Input: part model. Units: mm. Frame: model coordinates. A direction names the side the tool comes from. Give positions to 0.01 mm unless a question says otherwise; leave off trailing zeros. Write each loop counter-clockwise with the first axis right and the second up, starting at its lowest first coordinate (ties: lowest second). Pieces come first, ordered by that corner, then holes. Notation, with made-up numbers: (44.25, 87.5) -> (96.25, 87.5) arc R28 cw to (96.25, 122.5) -> close; hole circle Ø4 at (27, -24.5). An arc over 180 degrees is marked (long way). Return JSON: item names as keys, results as strings. Group by question number.
Item 1: Set-up query: faces 1 (the face through (-16, 16, -2)), 2 (the face through (0, 45, 0)), 3 (the face through (-12, 17, 4)), 4 (the face through (0, -12, 7)). Return all of +Z, -Z, +X, -X, +Y, -Y with unobstructed straight access to the full face (end or side cutting, diameter ignored); none if empty.
Item 2: Mould query, pull axis Z, two halves, no side actions, for faces 5 (the face through (16, 16, -2)), 6 (the face through (14.03, 21.27, 5)), 7 (the face through (0, 45, 7)), 8 (the face through (-14.028, 21.495, 3.72)). Classes: released by +Z, released by -Z, zero draft, split by the parting line, or undercut.
Item 3: Section A-A, the plane y = 0. Return loops of the section in (x, z), then the cut area to 3 significant figures.
Item 4: Section D-D, the plane y = 33. Return loops of the section in (x, z).
Item 5: Line query: line 1 (X direction, y = 0, z = 1.75); line 2 (Y direction, x = -4.5, z = 2.5); line 3 (Y direction, x = -15, z = 5.75). Output: solid intervals per line, ascending. Write a range as [from, to].
Item 6: Section C-C, the plane z = 6. Return loops of the section in (x, y).
Item 7: Section B-B, the plane x = -1. Return loops of the section in (y, z), then the cut area to 3 significant figures.
Item 8: Pin query (flat end, axial travel): P1, Ø1.5, axis at x = 7, y = 17.5, coming from the +Z side; P2, Ø4, axis at x = -11.5, y = 7, coming from the -Z side; P3, Ø2, axis at x = 8.5, y = 34.5, coming from the -Z side; P4, Ø6, axis at y = 16.5, z = 3.5, coming from the -X side. Return the tip coordinate at first contact, or that it passes through.
from build123d import *

# Parameters (mm, degrees)
F0_R          = 11
F1_DEPTH      = 7
F3_DEPTH      = 16
F3_DEPTH_BACK = 16
F4_R          = 5
F5_DEPTH      = 4
F6_R          = 5
F7_DEPTH      = 4


# Not quite as in the source:
# - a feature of the source that left no trace in its solid (it failed there, or was rolled back) is left out


with BuildPart() as f1:
    # F0 (on Top) → F1 (new body)
    with BuildSketch(Plane.XY):
        with BuildLine():
            ThreePointArc((13.2046790968, 10.5469991105), (14.5476279215, 16.7175814785), (13.1493192392, 22.8758548676))
            ThreePointArc((13.1493192392, 22.8758548676), (0, 49.5952677326), (-13.1493192392, 22.8758548676))
            ThreePointArc((-13.1493192392, 22.8758548676), (-14.5476279215, 16.7175814785), (-13.2046790968, 10.5469991105))
            ThreePointArc((-13.2046790968, 10.5469991105), (0, -16.8997852142), (13.2046790968, 10.5469991105))
        make_face()
        Circle(F0_R, mode=Mode.SUBTRACT)
        with Locations((0, 33)):
            Circle(F0_R, mode=Mode.SUBTRACT)
    extrude(amount=F1_DEPTH)

    # F2 (on Right) → F3 (join, two sides)
    with BuildSketch(Plane.YZ) as f3_sk:
        with BuildLine():
            ThreePointArc((9.306252715, 7), (14.7041684767, -4.2958315233), (24.5, 3.5))
            ThreePointArc((24.5, 3.5), (18.2958315233, 11.2958315233), (9.306252715, 7))
        make_face()
    extrude(amount=F3_DEPTH)
    extrude(f3_sk.sketch, amount=-F3_DEPTH_BACK)

    # F4 (on face) → F5 (cut)
    with BuildSketch(Plane.YZ.offset(16)):
        with Locations((16.5, 3.5)):
            Circle(F4_R)
    extrude(amount=-F5_DEPTH, mode=Mode.SUBTRACT)

    # F6 (on face) → F7 (cut)
    with BuildSketch(Plane(origin=(-16, 0, 0), x_dir=(0, -1, 0), z_dir=(-1, 0, 0))):
        with Locations((-16.5, 3.5)):
            Circle(F6_R)
    extrude(amount=-F7_DEPTH, mode=Mode.SUBTRACT)


solid = f1.part
Answer below:
{
 "1": {"face 1": "+Z, -Z, -X", "face 2": "-Z, +X, -X, +Y", "face 3": "-X", "face 4": "+Z, +X, -X, -Y"},
 "2": {"face 5": "zero draft", "face 6": "undercut", "face 7": "released by +Z", "face 8": "undercut"},
 "3": {"outline": "(-16.9, 0) -> (-11, 0) -> (-11, 7) -> (-16.9, 7) -> close; (11, 0) -> (16.9, 0) -> (16.9, 7) -> (11, 7) -> close", "area": "82.6 mm2"},
 "4": {"outline": "(-16.6, 0) -> (-11, 0) -> (-11, 7) -> (-16.6, 7) -> close; (11, 0) -> (16.6, 0) -> (16.6, 7) -> (11, 7) -> close"},
 "5": {"line 1": "x = [-16.9, -11], [11, 16.9]", "line 2": "y = [-16.29, -10.04], [8.56, 24.44], [43.04, 48.97]", "line 3": "y = [-7.78, 7.78], [8.82, 12.03], [20.97, 24.18], [25.9, 40.1]"},
 "6": {"outline": "(-16, 8.9) -> (-14.37, 8.9) arc R16.9 ccw (long way) to (14.37, 8.9) -> (16, 8.9) -> (16, 12.17) -> (12, 12.17) -> (12, 20.83) -> (16, 20.83) -> (16, 24.1) -> (14.01, 24.1) arc R16.6 ccw (long way) to (-14.01, 24.1) -> (-16, 24.1) -> (-16, 20.83) -> (-12, 20.83) -> (-12, 12.17) -> (-16, 12.17) -> close; hole (-6.46, 8.9) arc R11 ccw (long way) to (6.46, 8.9) -> close; hole (-6.46, 24.1) -> (6.46, 24.1) arc R11 ccw (long way) to start"},
 "7": {"outline": "(-16.87, 0) -> (-10.95, 0) -> (-10.95, 7) -> (-16.87, 7) -> close; circle Ø16 at (16.5, 3.5); (43.95, 0) -> (49.57, 0) -> (49.57, 7) -> (43.95, 7) -> close", "area": "282 mm2"},
 "8": {"P1": "stops at z = 11.5", "P2": "stops at z = 0", "P3": "passes through", "P4": "stops at x = -12"}
}
